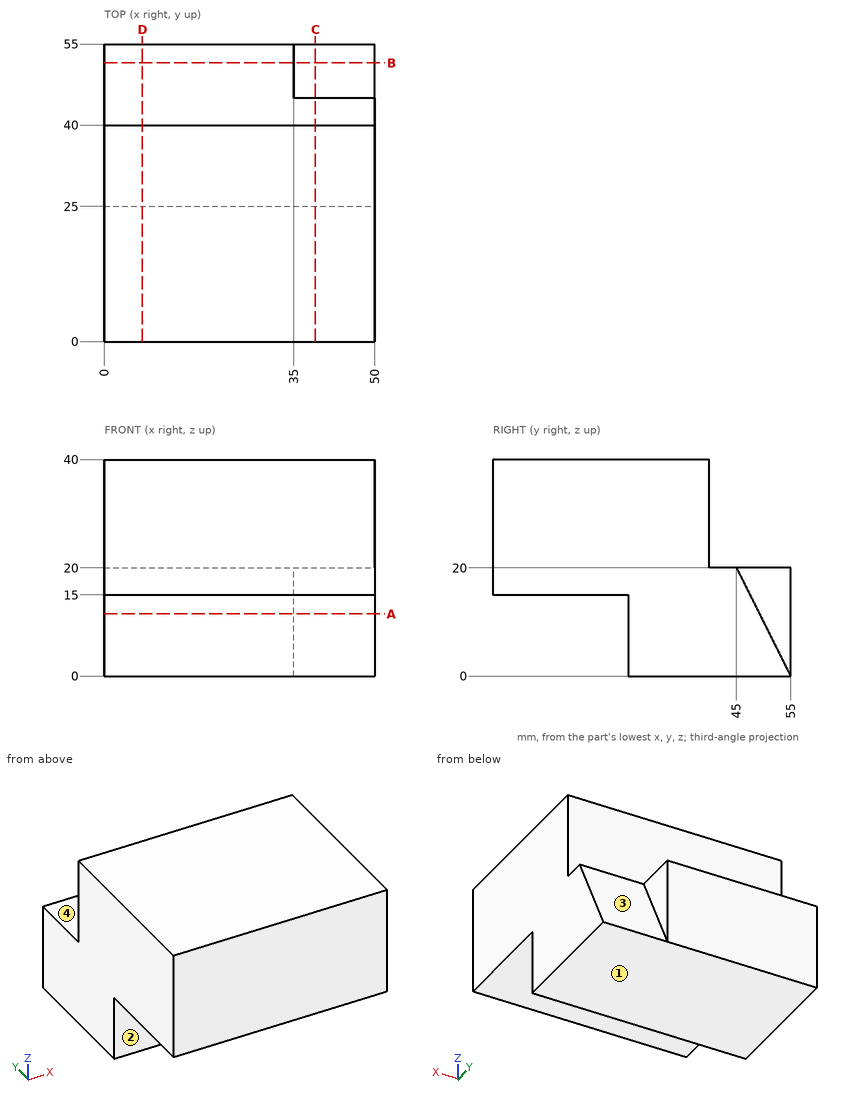
Drawing for the job (mm, zero at the part's lowest x, y, z). A direction names the side the tool comes from. Coordinates: 2 decimals unless noted, no trailing zeros. Order: outer loops, then holes, each group sorted by start corner. A loop starts at its lowest first (then second) coordinate and runs counter-clockwise, first axis right, second up. Notation, with made-up numbers: (18, -21.75) -> (25, -21.75) arc R13 cw to (25, 3.25) -> close; hole circle Ø4 at (60, 81). An arc over 180 degrees is marked (long way). One line per item, written item: value.
(1) Slice it at B-B, the plane y = 51.5. List the corners of the cut face in (x, z).
Checked values:
outline: (0, 0) -> (50, 0) -> (50, 7) -> (35, 7) -> (35, 20) -> (0, 20) -> close
(2) Tool access for the marked faces 1, 2, 3 and 4: list every direction of +Z, -Z, +X, -X, +Y, -Y with a clear straight run to the whole face (end or side of a thin tool).
Checked values:
face 1: -Z, +X, -X, +Y, -Y
face 2: -Z, +X, -X, -Y
face 3: +Z, +X, +Y
face 4: +Z, +X, -X, +Y
(3) Drop flat-ended pins along their axis: pin 1 Ø7.5 at (x, z) = (29, 9) entering from -Y; pin 2 Ø7.5 at (x, y) = (17, 50) entering from +Z; pin 3 Ø16 at (x, z) = (28.5, 28.5) entering from +Y. Give the stop position or say it passes through.
Checked values:
pin 1: y = 25
pin 2: z = 20
pin 3: y = 40
(4) Slice it at C-C, the plane x = 39. List the corners of the cut face in (y, z).
Checked values:
outline: (0, 15) -> (25, 15) -> (25, 0) -> (55, 0) -> (45, 20) -> (40, 20) -> (40, 40) -> (0, 40) -> close
(5) Slice it at D-D, the plane x = 7. List the corners of the cut face in (y, z).
Checked values:
outline: (0, 15) -> (25, 15) -> (25, 0) -> (55, 0) -> (55, 20) -> (40, 20) -> (40, 40) -> (0, 40) -> close
(6) Probe line 1 (Y direction, x = 6, z = 10.5); line 2 (Z direction, x = 34, y = 16.5); line 3 (Y direction, x = 9.5, z = 22). List the from-to ranges inside material, lowest first. Write a range as [from, to].
Checked values:
line 1: [25, 55]
line 2: [15, 40]
line 3: [0, 40]
(7) Slice it at A-A, the plane z = 11.5. List the corners of the cut face in (x, y), plus the area to 3 significant figures.
Checked values:
outline: (0, 25) -> (50, 25) -> (50, 49.25) -> (35, 49.25) -> (35, 55) -> (0, 55) -> close
area: 1,410 mm2
